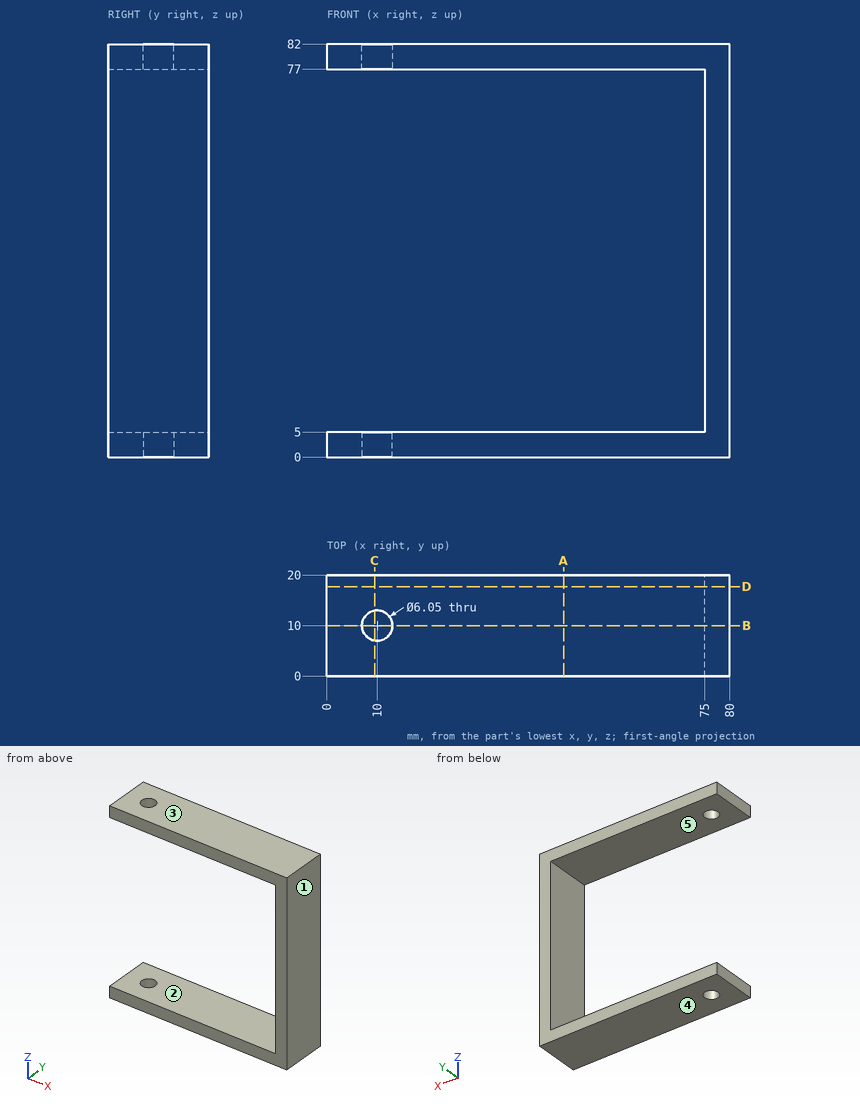
Geometry check sheet. Reference: drawing and pictorial views, mm from the part's lowest x, y, z. A direction names the side the tool comes from. Coordinates: 2 decimals unless noted, no trailing zeros. Order: outer loops, then holes, each group sorted by start corner. A loop starts at its lowest first (then second) coordinate and runs counter-clockwise, first axis right, second up.
1. Sectioned sample at B-B, the plane y = 10. Record the cut outline in (x, z) (3 decimals).
Results found:
outline: (0, 0) - (6.975, 0) - (6.975, 5) - (0, 5) - close; (0, 77) - (6.975, 77) - (6.975, 82) - (0, 82) - close; (13.025, 0) - (80, 0) - (80, 82) - (13.025, 82) - (13.025, 77) - (75, 77) - (75, 5) - (13.025, 5) - close
2. Sectioned sample at C-C, the plane x = 9.5. Record the cut outline in (y, z), and give its area (3 significant figures).
Results found:
outline: (0, 0) - (7.02, 0) - (7.02, 5) - (0, 5) - close; (0, 77) - (7.02, 77) - (7.02, 82) - (0, 82) - close; (12.98, 0) - (20, 0) - (20, 5) - (12.98, 5) - close; (12.98, 77) - (20, 77) - (20, 82) - (12.98, 82) - close
area: 140 mm2
3. Sectioned sample at D-D, the plane y = 17.75. Record the cut outline in (x, z), and give its area (3 significant figures).
Results found:
outline: (0, 0) - (80, 0) - (80, 82) - (0, 82) - (0, 77) - (75, 77) - (75, 5) - (0, 5) - close
area: 1,160 mm2
4. Set-up check for the marked faces 4 and 5: record each of +Z, -Z, +X, -X, +Y, -Y from which the full face is reachable in a straight line by a thin tool's end or side.
Results found:
face 4: -Z, +X, -X, +Y, -Y
face 5: -X, +Y, -Y
5. Go/stop test with flat-tipped pins: pin 1 Ø5 at (y, z) = (11, 34.5) entering from -X; pin 2 Ø12 at (x, y) = (49.5, 14) entering from -Z. Record where each tip stops, or that it passes through.
Results found:
pin 1: stops at x = 75
pin 2: stops at z = 0
6. Scan lines: line 1 (X direction, y = 10, z = 1.1) (3 decimals); line 2 (Z direction, x = 71.5, y = 17); line 3 (Y direction, x = 10, z = 79) (3 decimals). Record each from-to range of solid material in increasing order.
Results found:
line 1: x = 0 to 6.975, 13.025 to 80
line 2: z = 0 to 5, 77 to 82
line 3: y = 0 to 6.975, 13.025 to 20
7. Sectioned sample at A-A, the plane x = 47. Record the cut outline in (y, z), and give its area (3 significant figures).
Results found:
outline: (0, 0) - (20, 0) - (20, 5) - (0, 5) - close; (0, 77) - (20, 77) - (20, 82) - (0, 82) - close
area: 200 mm2
8. Release check for a two-part mould opening along Z. For the marked faces 1, 2 and 3 record: +Z half, -Z half, draft (parallel to the pull), parting line (faces both ways), or undercut.
Results found:
face 1: draft
face 2: undercut
face 3: +Z half
